Source: CAD feature listing. Evaluate the final solid. Frame: model axes, mm. Give positions to 0.01 mm unless a question says otherwise; leave off trailing zeros. Order: outer loops, then holes, each group sorted by start corner. A loop starts at its lowest first (then second) coordinate and runs counter-clockwise, first axis right, second up. Notation, with made-up numbers: (-36, -20) -> (-6, -20) arc R7 ccw to (-6, -15) -> close; hole circle Ø7 at (-7, 7). An arc over 180 degrees is marked (long way). Answer in a Markdown table with one row per item.
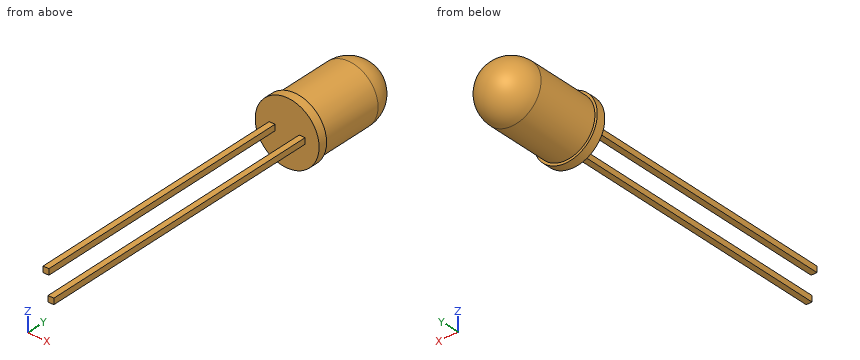
Autodesk Inventor part; units mm, degrees
ref_plane "YZ Plane" through (0, 0, 0) normal (1, 0, 0) x (0, 1, 0)
ref_plane "XZ Plane" through (0, 0, 0) normal (0, 1, 0) x (-1, 0, 0)
ref_plane "XY Plane" through (0, 0, 0) normal (0, 0, 1) x (1, 0, 0)
sketch "Sketch1" plane through (0, 0, 0) normal (0, 0, 1) x (1, 0, 0)
  line L0 (0, 0) -> (0, 8.7)
  arc A0 (2.5, 6.2) -> (0, 8.7) centre (0, 6.2) ccw
  line L1 (2.5, 6.2) -> (2.5, 0.7593)
  line L2 (2.5, 0.7593) -> (2.7, 0.7593)
  line L3 (2.7, 0.7593) -> (2.7, 0)
  line L4 (2.7, 0) -> (0, 0)
  dimension "d0" = 5
  dimension "d1" = 0.2
  dimension "d2" = 8.7
  dimension "d3" = 0.7593
revolve "Revolution1" add sketch "Sketch1" angle 360 about axis through (0, 0, 0) along (0, 1, 0)
sketch "Sketch2" plane through (0, 0, 0) normal (0, -1, 0) x (1, 0, 0)
  line L0 (-1.52, 0.25) -> (-1.02, 0.25)
  line L1 (-1.02, 0.25) -> (-1.02, -0.25)
  line L2 (-1.02, -0.25) -> (-1.52, -0.25)
  line L3 (-1.52, -0.25) -> (-1.52, 0.25)
  line L4 (1.02, 0.25) -> (1.52, 0.25)
  line L5 (1.52, 0.25) -> (1.52, -0.25)
  line L6 (1.52, -0.25) -> (1.02, -0.25)
  line L7 (1.02, -0.25) -> (1.02, 0.25)
  point P0 (0, 0)
  point P1 (1.02, 0)
  dimension "d5" = 2.54
  dimension "d6" = 1.02
  dimension "d7" = 1.02
  dimension "d8" = 0.5
extrude "Extrusion1" add sketch "Sketch2" along normal blind 25.4 contours L4 L5 L6 L7
extrude "Extrusion2" add sketch "Sketch2" along normal blind 22.86 contours L0 L1 L2 L3
properties part number "LED"
(1) First-contact query: pin 1 Ø1.5 at (y, z) = (-20, 0.5) entering from +X; pin 2 Ø1.5 at (x, y) = (-1.5, -6.5) entering from -Z; pin 3 Ø0.6 at (x, z) = (-1.5, 0) entering from -Y. Flat tips, straight axial feed; report the tip coordinate or a pass-through.
A:
| item | result |
|---|---|
| pin 1 | stops at x = 1.52 |
| pin 2 | stops at z = -0.25 |
| pin 3 | stops at y = -22.86 |
(2) Section query A-A (x = 0). Return the cut outline in (y, z).
A:
| item | result |
|---|---|
| outline | (0, -2.7) -> (0.76, -2.7) -> (0.76, -2.5) -> (6.2, -2.5) arc R2.5 ccw to (6.2, 2.5) -> (0.76, 2.5) -> (0.76, 2.7) -> (0, 2.7) -> close |
(3) Ray query, probe 1 along X at (y, z) = (-20.5, -0.2); probe 2 along Z at (x, y) = (1.35, -16); probe 3 along X at (y, z) = (1.5, 0.15). Return the intervals inside material, ascending.
A:
| item | result |
|---|---|
| probe 1 | x = -1.52 to -1.02, 1.02 to 1.52 |
| probe 2 | z = -0.25 to 0.25 |
| probe 3 | x = -2.5 to 2.5 |
(4) Section query B-B (z = -1.85). Return the cut outline in (x, y), plus the area to 3 significant figures.
A:
| item | result |
|---|---|
| outline | (-1.97, 0) -> (1.97, 0) -> (1.97, 0.76) -> (1.68, 0.76) -> (1.68, 6.2) arc R1.68 ccw to (-1.68, 6.2) -> (-1.68, 0.76) -> (-1.97, 0.76) -> close |
| area | 25.7 mm^2 |
(5) Section query C-C (y = 3.5). Return the cut outline in (x, z).
A:
| item | result |
|---|---|
| outline | circle Ø5 at (0, 0) |
